Geometry: see drawing. Coordinates: mm, zero at the bounding-box minimum. Round coordinates to 2 decimals unless told otherwise and drop trailing zeros. Loops run counter-clockwise (first coordinate to the right, second up) from the corner with the lowest first, then second, coordinate; pieces in that order, holes last.
(1) Section A-A, the plane x = 97. Return the cut outline in (y, z) (1 decimal).
(2) Section B-B, the plane y = 73. Return the cut outline in (x, z).
(3) Mould query, pull axis X, two halves, no side actions, for the marked faces 1, 2 and 3. Classes: pulls with the +X half, pulls with the -X half, needs draft (parallel to the pull), parting line crosses it, or undercut.
(4) Material intervals for probe 1 along X at (y, z) = (7, 10.25) (1 decimal); probe 2 along Y at (x, z) = (9.5, 11.25) (1 decimal); probe 3 along X at (y, z) = (14.5, 11.75) (1 decimal), sorted ascending.
(5) First-contact query: pin 1 Ø3.5 at (x, y) = (92.76, 13.72) entering from -Z; pin 2 Ø1.5 at (x, z) = (75.5, 9) entering from +Y; pin 3 Ø5 at (y, z) = (49.5, 11) entering from +X (1 decimal); pin 4 Ø6 at (x, z) = (42, 8.5) entering from +Y. Flat tips, straight axial feed; report the tip coordinate or a pass-through.
(6) Section C-C, the plane z = 4. Count the separate pieces of the cut face and the enclosed holes in it, plus the area to 3 significant figures.
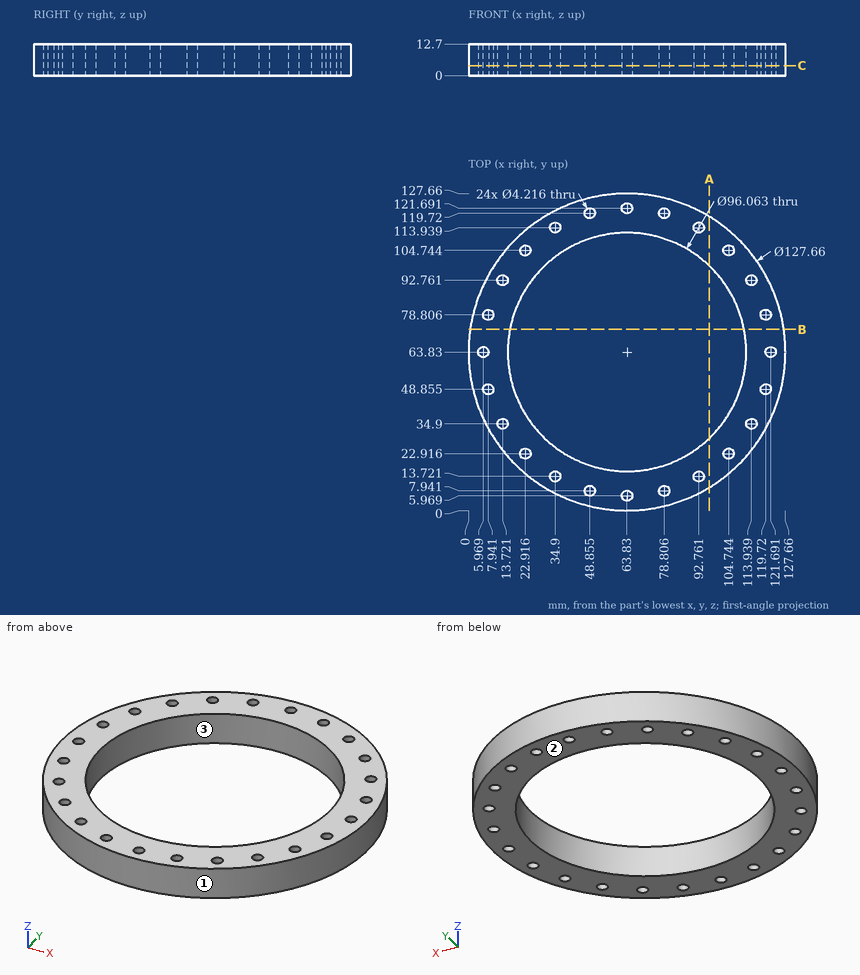
Output values:
1. outline: (9.3, 0) - (29.1, 0) - (29.1, 12.7) - (9.3, 12.7) - close; (98.6, 0) - (118.4, 0) - (118.4, 12.7) - (98.6, 12.7) - close
2. outline: (0.66, 0) - (16.68, 0) - (16.68, 12.7) - (0.66, 12.7) - close; (110.98, 0) - (127, 0) - (127, 12.7) - (110.98, 12.7) - close
3. face 1: parting line crosses it
3. face 2: needs draft
3. face 3: undercut
4. probe 1: x = 34.8 to 47, 50.7 to 62, 65.7 to 76.9, 80.7 to 92.9
4. probe 2: y = 30.3 to 47.4, 50.3 to 77.4, 80.2 to 97.3
4. probe 3: x = 23.3 to 32.9, 36.9 to 90.8, 94.7 to 104.3
5. pin 1: passes through
5. pin 2: stops at y = 126.72
5. pin 3: stops at x = 126.6
5. pin 4: stops at y = 124.82
6. separate pieces: 1
6. enclosed holes: 25
6. area: 5,220 mm2
